Part print with two shaded views. Sizes in mm from the minimum x, y, z corner. A direction names the side the tool comes from. Give positions to 0.01 mm unless a question says otherwise; leave off trailing zeros. Loops run counter-clockwise (first coordinate to the right, second up) from the corner with the lowest first, then second, coordinate; pieces in that order, holes last. Notation, with made-up numbers: M 52.5,26.5 L 102.5,26.5 A21 ccw 102.5,35.5 Z; hole C -15,-32 d6. An arc over 180 degrees is marked long. Answer in a Markdown table with one row per item.
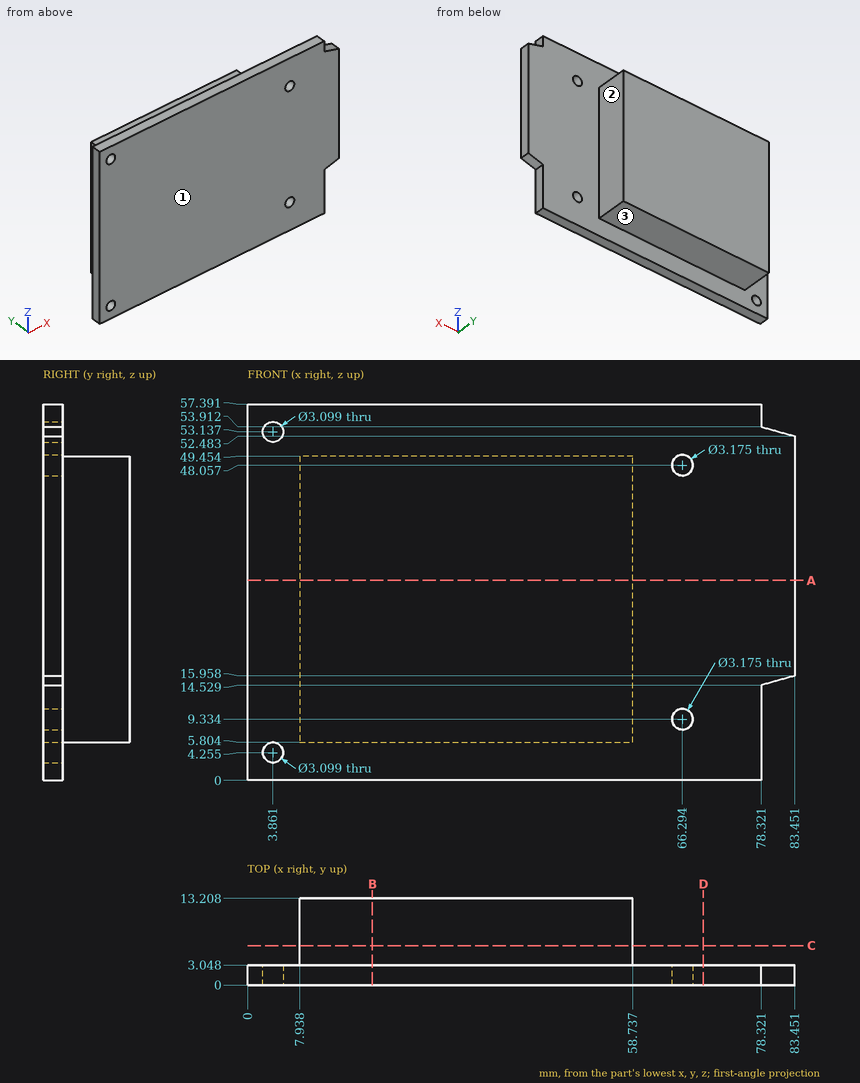
Q1. Probe probe 1 along X at (y, z) = (6, 24.5); probe 2 along Z at (x, y) = (24, 10); probe 3 along Y at (x, z) = (21.5, 52). List the from-to ranges inside material, lowest first.
Reported:
| item | result |
|---|---|
| probe 1 | 7.94 to 58.74 |
| probe 2 | 5.8 to 49.45 |
| probe 3 | 0 to 3.05 |
Q2. Saw through at A-A (z = 30.5). Give the cut face in (x, y).
Reported:
| item | result |
|---|---|
| outline | M 0,0 L 83.45,0 L 83.45,3.05 L 58.74,3.05 L 58.74,13.21 L 7.94,13.21 L 7.94,3.05 L 0,3.05 Z |
Q3. Saw through at D-D (x = 69.5). Give the cut face in (y, z), and give its area (3 significant figures).
Reported:
| item | result |
|---|---|
| outline | M 0,0 L 3.05,0 L 3.05,57.39 L 0,57.39 Z |
| area | 175 mm² |
Q4. Drop flat-ended pins along their axis: pin 1 (1.5 mm diameter, centred on y = 6, z = 32, fed in from -X); pin 2 (1 mm diameter, centred on x = 30.5, y = 9, fed in from +Z); pin 3 (2.5 mm diameter, centred on y = 1, z = 56, fed in from +X). Give the stop position or say it passes through.
Reported:
| item | result |
|---|---|
| pin 1 | x = 7.94 |
| pin 2 | z = 49.45 |
| pin 3 | x = 78.32 |
Q5. Saw through at C-C (y = 6). Give the cut face in (x, z), and give its area (3 significant figures).
Reported:
| item | result |
|---|---|
| outline | M 7.94,5.8 L 58.74,5.8 L 58.74,49.45 L 7.94,49.45 Z |
| area | 2,220 mm² |
Q6. 3-axis set-ups, long thin cutter, end or side, ignore diameter. For the marked faces 1, 2 and 3: which of +Z, -Z, +X, -X, +Y, -Y reach the whole face in a straight line?
Reported:
| item | result |
|---|---|
| face 1 | +Z, -Z, +X, -X, -Y |
| face 2 | +Z, -Z, +X, +Y |
| face 3 | -Z, +X, -X, +Y |
Q7. Saw through at B-B (x = 19). Give the cut face in (y, z).
Reported:
| item | result |
|---|---|
| outline | M 0,0 L 3.05,0 L 3.05,5.8 L 13.21,5.8 L 13.21,49.45 L 3.05,49.45 L 3.05,57.39 L 0,57.39 Z |
